The figure shows three views and two pictorial views of one solid part (mm, origin at its lowest corner). Answer the questions. A direction names the side the tool comes from. Round coordinates to 2 decimals unless told otherwise and drop trailing zeros. Write each loop counter-clockwise with the first axis right and the second up, starting at its lowest first coordinate (ties: lowest second). Pieces come first, ordered by that corner, then holes.
Item 1: Each of these flat-tipped pins is pushed along its axis until it touches: pin 1 (5 mm diameter, centred on x = 13.5, z = 3, fed in from -Y); pin 2 (6 mm diameter, centred on x = 22, z = 7, fed in from -Y). Where does it stop, or does it pass through?
Item 2: Find section C-C on y = 45. Give the vertices of the cut face in (x, z) (1 decimal).
Item 3: Find section D-D on x = 24. Give the vertices of the cut face in (y, z) (1 decimal), then the cut area to 3 significant figures.
Item 4: Find the intervals of material crossed by probe 1 along Z at (x, y) = (10.25, 66) (1 decimal); probe 2 along Y at (x, z) = (4.75, 23.5) (1 decimal), in increasing order.
Item 5: For a pull along X with two mould halves and no side action, classify the marked faces 1, 2 and 3 as +X half, -X half, draft (parallel to the pull), parting line (faces both ways), or undercut.
Item 6: Find section A-A on z = 16.75. Give the vertices of the cut face in (x, y) (1 decimal).
Item 7: A tool of negligible diameter and unlimited length cuts with its end or side. For the marked faces 4 and 5, from which of +Z, -Z, +X, -X, +Y, -Y can it reach the whole face along a straight path? Write none if from no direction.
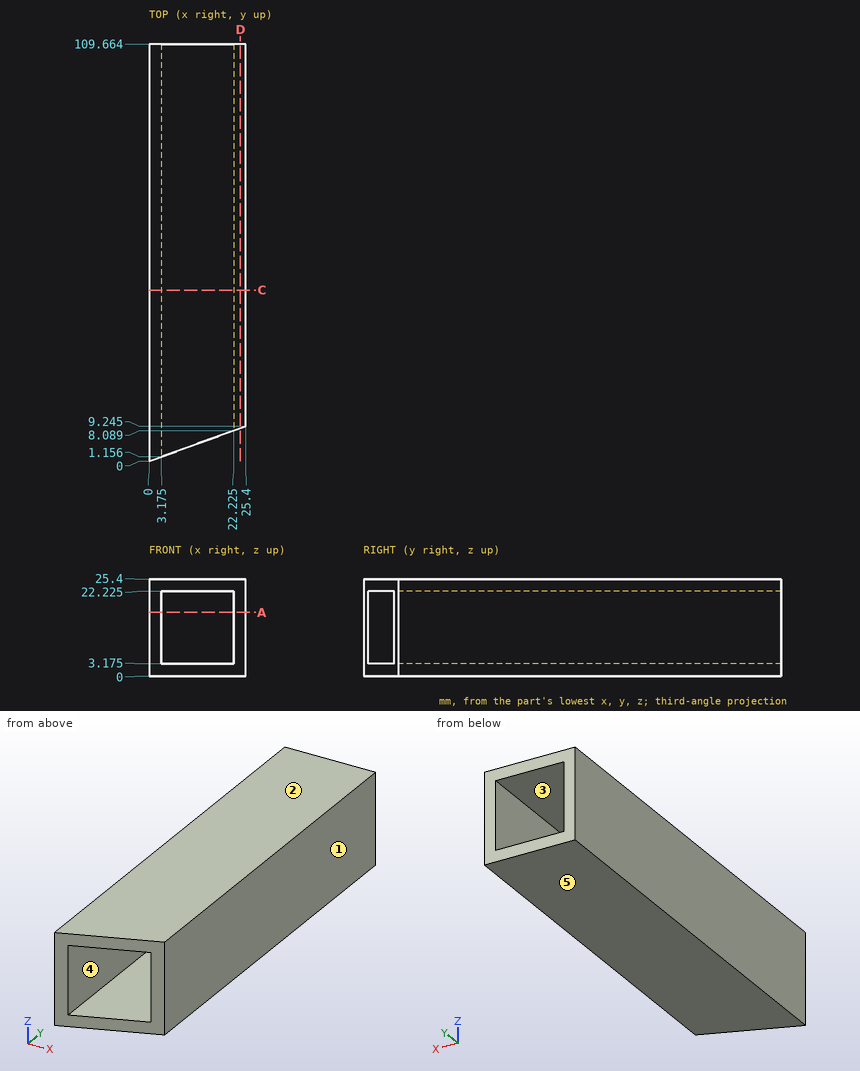
Check values:
1. pin 1: stops at y = 4
1. pin 2: stops at y = 8.09
2. outline: (0, 0) - (25.4, 0) - (25.4, 25.4) - (0, 25.4) - close; hole (3.2, 3.2) - (22.2, 3.2) - (22.2, 22.2) - (3.2, 22.2) - close
3. outline: (8.7, 0) - (109.7, 0) - (109.7, 25.4) - (8.7, 25.4) - close
3. area: 2,560 mm2
4. probe 1: z = 0 to 3.2, 22.2 to 25.4
4. probe 2: y = 1.7 to 109.7
5. face 1: +X half
5. face 2: draft
5. face 3: undercut
6. outline: (0, 0) - (3.2, 1.2) - (3.2, 109.7) - (0, 109.7) - close; (22.2, 8.1) - (25.4, 9.2) - (25.4, 109.7) - (22.2, 109.7) - close
7. face 4: +Y, -Y
7. face 5: -Z, +X, -X, +Y, -Y
